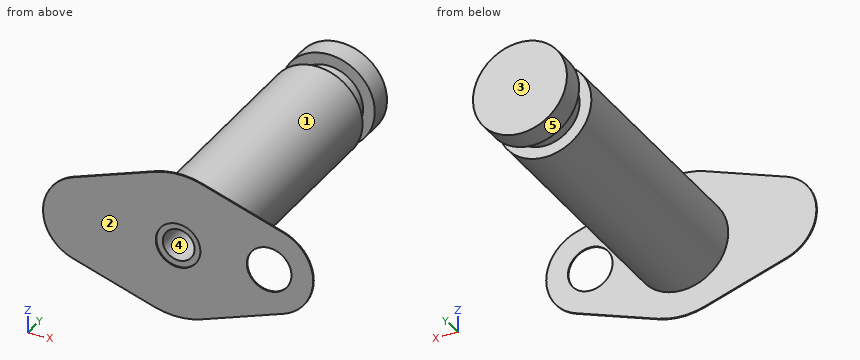
```python
from build123d import *

# Parameters (mm, degrees)
SKETCH1_R                      = 6.25
SKETCH1_R_2                    = 3.75
SKETCH1_R_3                    = 2.5
BOSS_EXTRUDE1_DEPTH            = 0.1
SKETCH2_R                      = 4
BOSS_EXTRUDE2_DEPTH            = 22.5
SKETCH3_R                      = 3
BOSS_EXTRUDE3_DEPTH            = 2
SKETCH4_R                      = 4
BOSS_EXTRUDE4_DEPTH            = 2
SKETCH6_W                      = 1.89865
SKETCH6_H                      = 0.1
F_6_CLEARANCE_HOLE1_AT_2_COUNT = 2
F_6_CLEARANCE_HOLE1_AT_2_PITCH = 7.75
F_6_32_TAPPED_HOLE2_D          = 2.7051
F_6_32_TAPPED_HOLE2_DEPTH      = 9.39
F_6_32_TAPPED_HOLE2_TIP        = 0.81269403


with BuildPart() as part:
    # Sketch1 → Boss-Extrude1 (new body)
    # profile 1 of 15: a face of its own
    with BuildSketch(Plane(origin=(0, 0, 0), x_dir=(1, 0, 0), z_dir=(0, 1, 0))):
        Circle(SKETCH1_R)
    # profile 2 of 15: a face of its own
    with BuildSketch(Plane(origin=(0, 0, 0), x_dir=(1, 0, 0), z_dir=(0, 1, 0))):
        with Locations((-7.75, 0)):
            Circle(SKETCH1_R_2)
        with Locations((-7.75, 0)):
            Circle(SKETCH1_R_3, mode=Mode.SUBTRACT)
    # profile 3 of 15: a face of its own
    with BuildSketch(Plane(origin=(0, 0, 0), x_dir=(1, 0, 0), z_dir=(0, 1, 0))):
        Circle(SKETCH1_R)
    # profile 4 of 15: a face of its own
    with BuildSketch(Plane(origin=(0, 0, 0), x_dir=(1, 0, 0), z_dir=(0, 1, 0))):
        with Locations((-7.75, 0)):
            Circle(SKETCH1_R_2)
        with Locations((-7.75, 0)):
            Circle(SKETCH1_R_3, mode=Mode.SUBTRACT)
    # profile 5 of 15: a face of its own
    with BuildSketch(Plane(origin=(0, 0, 0), x_dir=(1, 0, 0), z_dir=(0, 1, 0))):
        with Locations((7.75, 0)):
            Circle(SKETCH1_R_2)
    # profile 6 of 15: a face of its own
    with BuildSketch(Plane(origin=(0, 0, 0), x_dir=(1, 0, 0), z_dir=(0, 1, 0))):
        Circle(SKETCH1_R)
    # profile 7 of 15: a face of its own
    with BuildSketch(Plane(origin=(0, 0, 0), x_dir=(1, 0, 0), z_dir=(0, 1, 0))):
        with Locations((-7.75, 0)):
            Circle(SKETCH1_R_2)
    # profile 8 of 15: a face of its own
    with BuildSketch(Plane(origin=(0, 0, 0), x_dir=(1, 0, 0), z_dir=(0, 1, 0))):
        with BuildLine():
            ThreePointArc((-5.487903226, -2.990889196), (-7.15425073, -3.702375293), (-8.959677419, -3.54953244))
            Line((-8.959677419, -3.54953244), (-2.016129032, -5.9158874))
            ThreePointArc((-2.016129032, -5.9158874), (-4.026975125, -4.77974595), (-5.487903226, -2.990889196))
        make_face()
    # profile 9 of 15: a face of its own
    with BuildSketch(Plane(origin=(0, 0, 0), x_dir=(1, 0, 0), z_dir=(0, 1, 0))):
        with BuildLine():
            ThreePointArc((5.487903226, -2.990889196), (4.026975125, -4.77974595), (2.016129032, -5.9158874))
            Line((2.016129032, -5.9158874), (8.959677419, -3.54953244))
            ThreePointArc((8.959677419, -3.54953244), (7.15425073, -3.702375293), (5.487903226, -2.990889196))
        make_face()
    # profile 10 of 15: a face of its own
    with BuildSketch(Plane(origin=(0, 0, 0), x_dir=(1, 0, 0), z_dir=(0, 1, 0))):
        Circle(SKETCH1_R)
    # profile 11 of 15: a face of its own
    with BuildSketch(Plane(origin=(0, 0, 0), x_dir=(1, 0, 0), z_dir=(0, 1, 0))):
        with Locations((7.75, 0)):
            Circle(SKETCH1_R_2)
        with Locations((7.75, 0)):
            Circle(SKETCH1_R_3, mode=Mode.SUBTRACT)
    # profile 12 of 15: a face of its own
    with BuildSketch(Plane(origin=(0, 0, 0), x_dir=(1, 0, 0), z_dir=(0, 1, 0))):
        with Locations((7.75, 0)):
            Circle(SKETCH1_R_2)
        with Locations((7.75, 0)):
            Circle(SKETCH1_R_3, mode=Mode.SUBTRACT)
    # profile 13 of 15: a face of its own
    with BuildSketch(Plane(origin=(0, 0, 0), x_dir=(1, 0, 0), z_dir=(0, 1, 0))):
        Circle(SKETCH1_R)
    # profile 14 of 15: a face of its own
    with BuildSketch(Plane(origin=(0, 0, 0), x_dir=(1, 0, 0), z_dir=(0, 1, 0))):
        with BuildLine():
            Line((8.959677419, 3.54953244), (2.016129032, 5.9158874))
            ThreePointArc((2.016129032, 5.9158874), (4.026975125, 4.77974595), (5.487903226, 2.990889196))
            ThreePointArc((5.487903226, 2.990889196), (7.15425073, 3.702375293), (8.959677419, 3.54953244))
        make_face()
    # profile 15 of 15: a face of its own
    with BuildSketch(Plane(origin=(0, 0, 0), x_dir=(1, 0, 0), z_dir=(0, 1, 0))):
        with BuildLine():
            Line((-2.016129032, 5.9158874), (-8.959677419, 3.54953244))
            ThreePointArc((-8.959677419, 3.54953244), (-7.15425073, 3.702375293), (-5.487903226, 2.990889196))
            ThreePointArc((-5.487903226, 2.990889196), (-4.026975125, 4.77974595), (-2.016129032, 5.9158874))
        make_face()
    extrude(amount=BOSS_EXTRUDE1_DEPTH)

    # Sketch2 → Boss-Extrude2 (add)
    with BuildSketch(Plane(origin=(0, 0, 0), x_dir=(1, 0, 0), z_dir=(0, 1, 0))):
        with Locations(Location((0, 0, 0), (0, 0, 90))):
            Circle(SKETCH2_R)
    extrude(amount=BOSS_EXTRUDE2_DEPTH)

    # Sketch3 → Boss-Extrude3 (add)
    with BuildSketch(Plane(origin=(0, 22.5, 0), x_dir=(1, 0, 0), z_dir=(0, 1, 0))):
        with Locations(Location((0, 0, 0), (0, 0, 270))):
            Circle(SKETCH3_R)
    extrude(amount=BOSS_EXTRUDE3_DEPTH)

    # Sketch4 → Boss-Extrude4 (add)
    with BuildSketch(Plane(origin=(0, 24.5, 0), x_dir=(1, 0, 0), z_dir=(0, 1, 0))):
        with Locations(Location((0, 0, 0), (0, 0, 90))):
            Circle(SKETCH4_R)
    extrude(amount=BOSS_EXTRUDE4_DEPTH)

    # Sketch6 → #6 Clearance Hole1 (revolve, cut)
    with BuildSketch(Plane(origin=(7.75, 0.1, 0), x_dir=(0, 0, 1), z_dir=(1, 0, 0))):
        with Locations((0.949325, 0.05)):
            Rectangle(SKETCH6_W, SKETCH6_H)
    f_6_clearance_hole1 = revolve(axis=Axis((7.75, 6.45, 0), (0, -1, 0)), mode=Mode.SUBTRACT)

    # #6 Clearance Hole1 at 2: #6 Clearance Hole1 ×2
    with Locations(*[(-i * F_6_CLEARANCE_HOLE1_AT_2_PITCH, 0, 0) for i in range(1, F_6_CLEARANCE_HOLE1_AT_2_COUNT)]):
        add(f_6_clearance_hole1, mode=Mode.SUBTRACT)

    # #6-32 Tapped Hole2
    with Locations(Plane(origin=(0, 0.1, 0), x_dir=(-1, 0, 0), z_dir=(0, -1, 0))):
        with Locations((0, 0)):
            Hole(F_6_32_TAPPED_HOLE2_D / 2, depth=F_6_32_TAPPED_HOLE2_DEPTH)
            with Locations((0, 0, -(F_6_32_TAPPED_HOLE2_DEPTH + F_6_32_TAPPED_HOLE2_TIP / 2))):  # 118° drill point
                Cone(0, F_6_32_TAPPED_HOLE2_D / 2, F_6_32_TAPPED_HOLE2_TIP, mode=Mode.SUBTRACT)


solid = part.part
```
CAD build for the part. Positions are in the model's coordinates, mm. Face numbers are marked on the shaded views. A direction names the side the tool comes from. Round coordinates to 2 decimals unless told otherwise and drop trailing zeros. Loops run counter-clockwise (first coordinate to the right, second up) from the corner with the lowest first, then second, coordinate; pieces in that order, holes last. Notation, with made-up numbers: M -7,-17.75 L 34,-17.75 A16 cw 34,-10.75 Z; hole C -2.5,50 d2. An arc over 180 degrees is marked long. Return JSON: item names as keys, results as strings. Group by question number.
(1) Saw through at C-C, the plane z = -2.5. List the corners of the cut face in (x, y).
(2) Drop flat-ended pins along their axis: P1, Ø8, axis at x = -2, y = 19, coming from the +Z side; P2, Ø6, axis at x = -7.5, y = 20, coming from the +Z side; P3, Ø5, axis at x = 3.5, y = 7.5, coming from the +Z side; P4, Ø1.5, axis at y = 22.5, z = -1, coming from the +X side. Give the stop position or say it passes through.
(3) Saw through at B-B, the plane y = 15.5. List the corners of the cut face in (x, z), and give its area (3 significant figures).
(4) Tool access for the marked faces 1 and 2: list every direction of +Z, -Z, +X, -X, +Y, -Y with a clear straight run to the whole face (end or side of a thin tool).
(5) Saw through at D-D, the plane x = 7.75. List the corners of the cut face in (y, z).
(6) Wall check: probe 1 along Y at (x, z) = (3.25, -2); probe 2 along Y at (x, z) = (1.25, -1.25); probe 3 along Z at (x, y) = (7.75, 0.05). Give the ranges that are in metal, low to high. Write a range as [from, to].
(7) Saw through at A-A, the plane x = -3.5. List the corners of the cut face in (y, z).
(8) Mould opens along Z. For the marked faces 3, 4 and 5 say: +Z half, -Z half, draft (parallel to the pull), parting line (faces both ways), or undercut.
Answer list:
{
 "1": {"outline": "M -10.55,0 L 10.55,0 L 10.55,0.1 L 3.12,0.1 L 3.12,22.5 L 1.66,22.5 L 1.66,24.5 L 3.12,24.5 L 3.12,26.5 L -3.12,26.5 L -3.12,24.5 L -1.66,24.5 L -1.66,22.5 L -3.12,22.5 L -3.12,0.1 L -10.55,0.1 Z"},
 "2": {"P1": "z = 4", "P2": "through", "P3": "z = 3.87", "P4": "x = 3.99"},
 "3": {"outline": "C 0,0 d8", "area": "50.3 mm2"},
 "4": {"face 1": "+Y", "face 2": "+Z, -Z, +X, -X, -Y"},
 "5": {"outline": "M 0,-3.96 L 0.1,-3.96 L 0.1,-1.9 L 0,-1.9 Z; M 0,1.9 L 0.1,1.9 L 0.1,3.96 L 0,3.96 Z"},
 "6": {"probe 1": "[0, 22.5], [24.5, 26.5]", "probe 2": "[0.1, 26.5]", "probe 3": "[-3.96, -1.9], [1.9, 3.96]"},
 "7": {"outline": "M 0,-5.41 L 0.1,-5.41 L 0.1,-1.94 L 22.5,-1.94 L 22.5,1.94 L 0.1,1.94 L 0.1,5.41 L 0,5.41 Z; M 24.5,-1.94 L 26.5,-1.94 L 26.5,1.94 L 24.5,1.94 Z"},
 "8": {"face 3": "draft", "face 4": "undercut", "face 5": "parting line"}
}
